Part model, mm, in its own coordinate system. Face numbers are marked on the shaded views. A direction names the side the tool comes from. Give positions to 0.01 mm unless a question says otherwise; leave off trailing zeros. Order: outer loops, then holes, each group sorted by start corner. A loop starts at its lowest first (then second) coordinate and runs counter-clockwise, first axis right, second up. Notation, with made-up numbers: (-4.5, -6) -> (53.5, -6) arc R22 cw to (53.5, 33) -> close; hole circle Ø9 at (62, 29). An arc over 180 degrees is marked (long way). Write item = value, one per line. Start each with the question number.
(1) Which spindle directions (+Z, -Z, +X, -X, +Y, -Y) get a long thin tool onto all of the face, cutting with end or side? Do the marked faces 1, 2 and 3. Say none if no direction does.
(2) Saw through at A-A, the plane x = 0. State how many separate pieces and enclosed holes the cut face has, then the cut area to 3 significant figures.
(3) Saw through at B-B, the plane y = -65. List the corners of the cut face in (x, z).
(4) Flat gauge pins, fed straight in: pin 1 (1.5 mm diameter, centred on y = -56, z = 6.5, fed in from -X); pin 2 (3 mm diameter, centred on y = -15, z = 4.5, fed in from -X); pin 3 (13 mm diameter, centred on x = -15.5, y = 26.85, fed in from -Z); pin 4 (5 mm diameter, centred on y = -13, z = 8, fed in from +X). Where does each tip first touch, or does it go through?
(5) Two-plate mould, pull along X, no slides. Class the marked faces 4, 5 and 6: pulls with the +X half, pulls with the -X half, needs draft (parallel to the pull), parting line crosses it, or undercut.
(6) Saw through at D-D, the plane x = -52. List the corners of the cut face in (y, z), then the cut area to 3 significant figures.
(7) Probe line 1 along Y through (x, z) = (0, 9.75); line 2 along X through (y, z) = (-26.5, 18.25); line 3 along Y through (x, z) = (15.5, 16). List the from-to ranges inside material, lowest first. Write a range as from..to.
from build123d import *

# Parameters (mm, degrees)
CROQUIS1_R                = 15
CROQUIS1_R_2              = 8
SALIENTE_EXTRUIR1_DEPTH   = 20
SALIENTE_EXTRUIR1_2_DEPTH = 20
SALIENTE_EXTRUIR1_3_DEPTH = 20
CROQUIS1_R_3              = 20
CROQUIS1_R_4              = 4
SALIENTE_EXTRUIR1_4_DEPTH = 20
SALIENTE_EXTRUIR2_DEPTH   = 10
CORTAR_EXTRUIR1_START     = -10
CROQUIS3_R                = 8
CORTAR_EXTRUIR1_DEPTH     = 10


with BuildPart() as part:
    # Croquis1 → Saliente-Extruir1 (new body)
    with BuildSketch(Plane.XY):
        with Locations((0, -82.97)):
            Circle(CROQUIS1_R)
        with Locations((0, -82.97)):
            Circle(CROQUIS1_R_2, mode=Mode.SUBTRACT)
    extrude(amount=SALIENTE_EXTRUIR1_DEPTH)



with BuildPart() as body_2:
    # Croquis1 → Saliente-Extruir1 2 (new body)
    with BuildSketch(Plane.XY):
        with Locations((55, -65)):
            Circle(CROQUIS1_R)
        with Locations((55, -65)):
            Circle(CROQUIS1_R_2, mode=Mode.SUBTRACT)
    extrude(amount=SALIENTE_EXTRUIR1_2_DEPTH)


with BuildPart() as body_3:
    # Croquis1 → Saliente-Extruir1 3 (new body)
    with BuildSketch(Plane.XY):
        with Locations(Location((-55, -65, 0), (0, 0, 180))):
            Circle(CROQUIS1_R)
        with Locations(Location((-55, -65, 0), (0, 0, 180))):
            Circle(CROQUIS1_R_2, mode=Mode.SUBTRACT)
    extrude(amount=SALIENTE_EXTRUIR1_3_DEPTH)


with BuildPart() as body_4:
    # Croquis1 → Saliente-Extruir1 4 (new body)
    with BuildSketch(Plane.XY):
        with BuildLine():
            ThreePointArc((-21.854157167, 21.986264223), (-26.846787517, 15.5), (-29.967741935, 7.933123174))
            ThreePointArc((-29.967741935, 7.933123174), (-39, 0), (-29.967741935, -7.933123174))
            ThreePointArc((-29.967741935, -7.933123174), (-26.846787517, -15.5), (-21.854157167, -21.986264223))
            ThreePointArc((-21.854157167, -21.986264223), (-19.5, -33.774990748), (-8.113584768, -29.919387397))
            ThreePointArc((-8.113584768, -29.919387397), (0, -31), (8.113584768, -29.919387397))
            ThreePointArc((8.113584768, -29.919387397), (19.5, -33.774990748), (21.854157167, -21.986264223))
            ThreePointArc((21.854157167, -21.986264223), (26.846787517, -15.5), (29.967741935, -7.933123174))
            ThreePointArc((29.967741935, -7.933123174), (39, 0), (29.967741935, 7.933123174))
            ThreePointArc((29.967741935, 7.933123174), (26.846787517, 15.5), (21.854157167, 21.986264223))
            ThreePointArc((21.854157167, 21.986264223), (19.5, 33.774990748), (8.113584768, 29.919387397))
            ThreePointArc((8.113584768, 29.919387397), (0, 31), (-8.113584768, 29.919387397))
            ThreePointArc((-8.113584768, 29.919387397), (-19.5, 33.774990748), (-21.854157167, 21.986264223))
        make_face()
        Circle(CROQUIS1_R_3, mode=Mode.SUBTRACT)
        with Locations((31, 0)):
            Circle(CROQUIS1_R_4, mode=Mode.SUBTRACT)
        with Locations((15.5, -26.846787517)):
            Circle(CROQUIS1_R_4, mode=Mode.SUBTRACT)
        with Locations((-15.5, -26.846787517)):
            Circle(CROQUIS1_R_4, mode=Mode.SUBTRACT)
        with Locations((-31, 0)):
            Circle(CROQUIS1_R_4, mode=Mode.SUBTRACT)
        with Locations((-15.5, 26.846787517)):
            Circle(CROQUIS1_R_4, mode=Mode.SUBTRACT)
        with Locations((15.5, 26.846787517)):
            Circle(CROQUIS1_R_4, mode=Mode.SUBTRACT)
    extrude(amount=SALIENTE_EXTRUIR1_4_DEPTH)


with BuildPart() as part_1:
    add(part.part)

    add(body_2.part)  # Saliente-Extruir2 merges body 2

    add(body_3.part)  # Saliente-Extruir2 merges body 3

    add(body_4.part)  # Saliente-Extruir2 merges body 4
    # Croquis2 → Saliente-Extruir2 (add)
    with BuildSketch(Plane.XY):
        with BuildLine():
            Line((-39, 0), (-39, -32.071476789))
            ThreePointArc((-39, -32.071476789), (-44.036846437, -44.559737265), (-56.328516633, -50.058947709))
            ThreePointArc((-56.328516633, -50.058947709), (-69.988497958, -64.412693478), (-57.493543192, -79.791289408))
            ThreePointArc((-57.493543192, -79.791289408), (0, -97.97141107), (57.493543192, -79.791289408))
            ThreePointArc((57.493543192, -79.791289408), (69.988497958, -64.412693478), (56.328516633, -50.058947709))
            ThreePointArc((56.328516633, -50.058947709), (44.036846437, -44.559737265), (39, -32.071476789))
            Line((39, -32.071476789), (39, 0))
            ThreePointArc((39, 0), (36.279296141, -6.01074307), (29.967741935, -7.933123174))
            ThreePointArc((29.967741935, -7.933123174), (26.846787517, -15.5), (21.854157167, -21.986264223))
            ThreePointArc((21.854157167, -21.986264223), (19.5, -33.774990748), (8.113584768, -29.919387397))
            ThreePointArc((8.113584768, -29.919387397), (0, -31), (-8.113584768, -29.919387397))
            ThreePointArc((-8.113584768, -29.919387397), (-19.5, -33.774990748), (-21.854157167, -21.986264223))
            ThreePointArc((-21.854157167, -21.986264223), (-26.846787517, -15.5), (-29.967741935, -7.933123174))
            ThreePointArc((-29.967741935, -7.933123174), (-36.27929614, -6.01074307), (-39, 0))
        make_face()
    extrude(amount=SALIENTE_EXTRUIR2_DEPTH)

    # Croquis3 → Cortar-Extruir1 (cut)
    with BuildSketch(Plane.XY.offset(10).offset(CORTAR_EXTRUIR1_START)):
        with Locations(Location((-55, -65, 0), (0, 0, 180))):
            Circle(CROQUIS3_R)
        with Locations((0, -82.97)):
            Circle(CROQUIS3_R)
        with Locations((55, -65)):
            Circle(CROQUIS3_R)
    extrude(amount=CORTAR_EXTRUIR1_DEPTH, mode=Mode.SUBTRACT)


solid = part_1.part
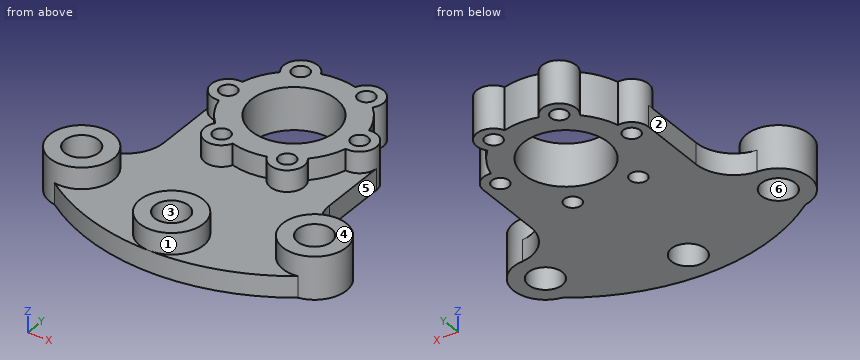
Results list:
q1.face_1 = +Z
q1.face_2 = +Z, -Z, -X, +Y
q1.face_3 = +Z, -Z
q2.separate_pieces = 3
q2.enclosed_holes = 0
q2.area = 1,090 mm^2
q3.outline = (-70, 0) -> (-63, 0) -> (-63, 20) -> (-70, 20) -> close; (-47, 0) -> (47, 0) -> (47, 20) -> (40, 20) -> (40, 10) -> (-40, 10) -> (-40, 20) -> (-47, 20) -> close; (63, 0) -> (70, 0) -> (70, 20) -> (63, 20) -> close
q4.pin_1 = -67.53
q4.pin_2 = -39
q4.pin_3 = 0
q4.pin_4 = 39
q5.face_4 = needs draft
q5.face_5 = pulls with the +X half
q5.face_6 = undercut
q6.outline = (-83.39, 0) -> (-72.42, 0) -> (-72.42, 20) -> (-79.7, 20) -> (-79.7, 10) -> (-83.39, 10) -> close; (-57.58, 0) -> (-49.36, 0) -> (-49.36, 10) -> (-50.3, 10) -> (-50.3, 20) -> (-57.58, 20) -> close
q6.area = 338 mm^2
q7.line_1 = -97.97..-90.97, -74.97..-20, 20..31
q7.line_2 = -23.49..-19.48, -11.52..11.52, 19.48..23.49
q7.line_3 = -34.85..-30.85, -22.85..-12.64, 12.64..22.85, 30.85..34.85
